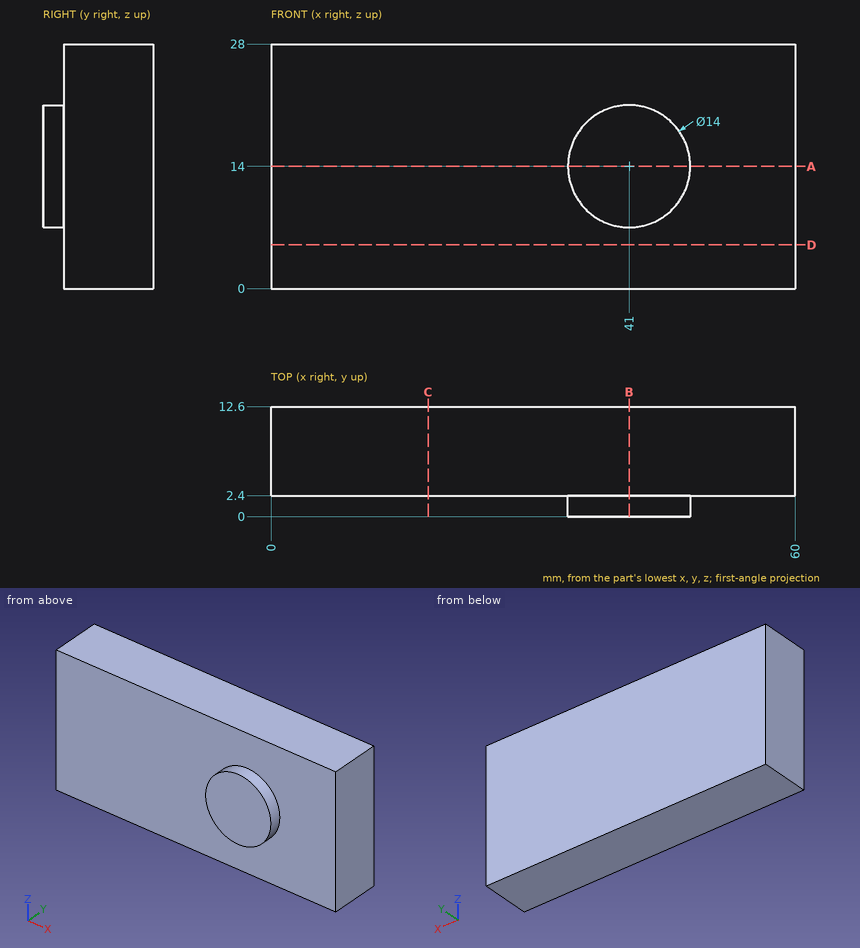
Study the drawing (mm; zero at the part's minimum x, y, z) and answer. Give positions to 0.01 mm unless a question says otherwise; leave off trailing zeros. Order: outer loops, then holes, each group sorted by start corner. A loop starts at its lowest first (then second) coordinate and runs counter-clockwise, first axis right, second up. Notation, with made-up numbers: (5.25, 7) - (41.25, 7) arc R9 ccw to (41.25, 23) - close; hole circle Ø1 at (80, -40). An arc over 180 degrees is marked (long way). Answer in a Markdown table with one row per item. Add a question column.
Q1. The part is cut by section A-A (z = 14). Determine the outline of the cut face in (x, y).
Q2. Find the intervals of material crossed by line 1 along Y through (x, z) = (54, 19.75), in increasing order. Write a range as [from, to].
Q3. The part is cut by section C-C (x = 18). Determine the outline of the cut face in (y, z).
Q4. The part is cut by section D-D (z = 5). Determine the outline of the cut face in (x, y), then the cut area to 3 significant figures.
Q5. Given P1, Ø6, axis at x = 51, z = 12.5, coming from the -Y side, flat-ended and moving along its own axis, determine where the tip first touches the part or whether it passes through.
Q6. The part is cut by section B-B (x = 41). Determine the outline of the cut face in (y, z), then the cut area to 3 significant figures.
Determined:
| question | item | result |
|---|---|---|
| 1 | outline | (0, 2.4) - (34, 2.4) - (34, 0) - (48, 0) - (48, 2.4) - (60, 2.4) - (60, 12.6) - (0, 12.6) - close |
| 2 | line 1 | y = [2.4, 12.6] |
| 3 | outline | (2.4, 0) - (12.6, 0) - (12.6, 28) - (2.4, 28) - close |
| 4 | outline | (0, 2.4) - (60, 2.4) - (60, 12.6) - (0, 12.6) - close |
| 4 | area | 612 mm² |
| 5 | P1 | stops at y = 2.4 |
| 6 | outline | (0, 7) - (2.4, 7) - (2.4, 0) - (12.6, 0) - (12.6, 28) - (2.4, 28) - (2.4, 21) - (0, 21) - close |
| 6 | area | 319 mm² |
